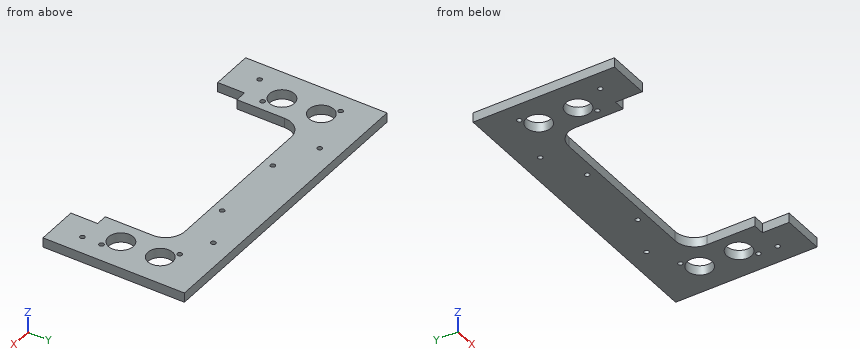
from build123d import *

# Parameters (mm, degrees)
F1_DEPTH = 6.35
F2_R     = 1.5875
F2_R_2   = 8.255
F3_DEPTH = 6.35


with BuildPart() as f1:
    # F0 (on Top) → F1 (new body)
    with BuildSketch(Plane.XY):
        with BuildLine():
            Line((0, 93.98), (0, 0))
            Line((0, 0), (27.94, 0))
            Line((27.94, 0), (27.94, 17.78))
            Line((27.94, 17.78), (35.56, 17.78))
            Line((35.56, 17.78), (35.56, 49.53))
            ThreePointArc((35.56, 49.53), (39.279744, 58.510256), (48.26, 62.23))
            Line((48.26, 62.23), (154.94, 62.23))
            ThreePointArc((154.94, 62.23), (163.920256, 58.510256), (167.64, 49.53))
            Line((167.64, 49.53), (167.64, 17.78))
            Line((167.64, 17.78), (175.26, 17.78))
            Line((175.26, 17.78), (175.26, 0))
            Line((175.26, 0), (203.2, 0))
            Line((203.2, 0), (203.2, 93.98))
            Line((203.2, 93.98), (0, 93.98))
        make_face()
    extrude(amount=F1_DEPTH)

    # F2 (on face) → F3 (cut)
    with BuildSketch(Plane.XY.offset(6.35)):
        with Locations((12.7, 17.78)):
            Circle(F2_R)
        with Locations((28.956, 30.48)):
            Circle(F2_R)
        with Locations((20.828, 37.973)):
            Circle(F2_R_2)
        with Locations((20.828, 64.135)):
            Circle(F2_R_2)
        with Locations((12.7, 71.628)):
            Circle(F2_R)
        with Locations((48.26, 81.28)):
            Circle(F2_R)
        with Locations((76.2, 68.58)):
            Circle(F2_R)
        with Locations((127, 68.58)):
            Circle(F2_R)
        with Locations((154.94, 81.28)):
            Circle(F2_R)
        with Locations((174.244, 71.628)):
            Circle(F2_R)
        with Locations((182.372, 64.135)):
            Circle(F2_R_2)
        with Locations((182.372, 37.973)):
            Circle(F2_R_2)
        with Locations((190.5, 30.48)):
            Circle(F2_R)
        with Locations((190.5, 17.78)):
            Circle(F2_R)
    extrude(amount=-F3_DEPTH, mode=Mode.SUBTRACT)


solid = f1.part
Input: part model. Units: mm. Frame: model coordinates. Give positions to 0.01 mm unless a question says otherwise; leave off trailing zeros. Write each loop counter-clockwise with the first axis right and the second up, starting at its lowest first coordinate (ties: lowest second). Pieces come first, ordered by that corner, then holes. Notation, with made-up numbers: M 62,22 L 116,22 A25 ccw 116,58 Z; hole C 87,-5.75 d6. An arc over 180 degrees is marked long. Write item = value, one per line. Start each with the question number.
1) First-contact query: pin 1 Ø5 at (x, y) = (150.5, 58) entering from +Z. Flat tip, straight axial feed; report the tip coordinate or a pass-through.
2) Cut plane C-C on z = 3. Count the separate pieces of the cut face and the enclosed holes in it, then the cut area to 3 significant figures.
3) Cut plane A-A on y = 8.5. Return the cut outline in (x, z).
4) Material intervals for line 1 along X through (y, z) = (81.28, 1.5); line 2 along X through (y, z) = (15, 2.75); line 3 along Y through (x, z) = (175.5, 2), sorted ascending. Write a range as [from, to].
5) Cut plane B-B on x = 21.5. Return the cut outline in (y, z), then the cut area to 3 significant figures.
6) Cut plane D-D on x = 148.5. Return the cut outline in (y, z), then the cut area to 3 significant figures.
Solved:
q1.pin_1 = through
q2.separate_pieces = 1
q2.enclosed_holes = 14
q2.area = 9,740 mm2
q3.outline = M 0,0 L 27.94,0 L 27.94,6.35 L 0,6.35 Z; M 175.26,0 L 203.2,0 L 203.2,6.35 L 175.26,6.35 Z
q4.line_1 = [0, 46.67], [49.85, 153.35], [156.53, 203.2]
q4.line_2 = [0, 27.94], [175.26, 203.2]
q4.line_3 = [0, 33.4], [42.55, 59.56], [68.71, 70.66], [72.6, 93.98]
q5.outline = M 0,0 L 29.75,0 L 29.75,6.35 L 0,6.35 Z; M 46.2,0 L 55.91,0 L 55.91,6.35 L 46.2,6.35 Z; M 72.36,0 L 93.98,0 L 93.98,6.35 L 72.36,6.35 Z
q5.area = 388 mm2
q6.outline = M 62.23,0 L 93.98,0 L 93.98,6.35 L 62.23,6.35 Z
q6.area = 202 mm2
